from build123d import *

# Parameters (mm, degrees)
F1_DEPTH = 25
F3_DEPTH = 24


with BuildPart() as f1:
    # F0 (on Right) → F1 (new body)
    with BuildSketch(Plane.YZ):
        Polygon((0, 30.708406), (0, 0), (6.495294, 0), (6.495294, 8.168684), (15.046757, 8.168684), (15.046757, 14.439756), (6.637818, 14.439756), (6.637818, 21.7085), (46.972219, 21.7085), (46.972219, 0), (57.595324, 0), (57.595324, 30.708406), align=None)
    extrude(amount=F1_DEPTH)

    # F2 (on face) → F3 (cut)
    with BuildSketch(Plane(origin=(0, 0, 0), x_dir=(0, -1, 0), z_dir=(-1, 0, 0))):
        Polygon((-53.99179, -2.160003), (-53.99179, 28.144645), (-3.114748, 28.144645), (-3.114748, 0), (2.5671, 0), (2.5671, 33.474556), (-65.965217, 33.474556), (-65.965217, -2.160003), align=None)
    extrude(amount=-F3_DEPTH, mode=Mode.SUBTRACT)


solid = f1.part
Check sheet for the modelled part. Datum: model origin and axes. Units: mm. A direction names the side the tool comes from. Round coordinates to 2 decimals unless told otherwise and drop trailing zeros. Write each loop counter-clockwise with the first axis right and the second up, starting at its lowest first coordinate (ties: lowest second). Pieces come first, ordered by that corner, then holes. Notation, with made-up numbers: (-30.5, -33) - (-3.5, -33) arc R6 ccw to (-3.5, -25) - close; hole circle Ø5 at (-14, 78). An arc over 180 degrees is marked (long way). Return JSON: item names as keys, results as strings.
Q1. Depth check by flat-ended pin: P1, Ø4.5, axis at x = 17, y = 10.5, coming from the -Z side; P2, Ø8, axis at x = 17.5, z = 17.5, coming from the +Y side; P3, Ø11, axis at x = 18, z = 14, coming from the -Y side. Enter the tip coordinate at first touch or a pass-through.
Returned:
{"P1": "stops at z = 8.17", "P2": "stops at y = 53.99", "P3": "stops at y = 3.11"}
Q2. Cross-section at B-B (z = 5.5). Record the boundary of the cut face in (x, y).
Returned:
{"outline": "(0, 3.11) - (24, 3.11) - (24, 0) - (25, 0) - (25, 6.5) - (0, 6.5) - close; (0, 46.97) - (25, 46.97) - (25, 57.6) - (24, 57.6) - (24, 53.99) - (0, 53.99) - close"}
Q3. Cross-section at C-C (x = 3.5). Record the boundary of the cut face in (y, z).
Returned:
{"outline": "(3.11, 0) - (6.5, 0) - (6.5, 8.17) - (15.05, 8.17) - (15.05, 14.44) - (6.64, 14.44) - (6.64, 21.71) - (46.97, 21.71) - (46.97, 0) - (53.99, 0) - (53.99, 28.14) - (3.11, 28.14) - close"}
Q4. Draft check along Y on faces 1 (the flat face through (24, 35, 29)), 2 (the flat face through (12, 3.115, 14)), 3 (the flat face through (12, 27, 21.708)), 4 (the flat face through (12, 11, 8.169)). Enter one of: released by +Y, released by -Y, zero draft, split by the parting line, or undercut.
Returned:
{"face 1": "zero draft", "face 2": "released by -Y", "face 3": "undercut", "face 4": "undercut"}
Q5. Scan lines: L1, parallel to Y at x = 5.5, z = 21.5; L2, parallel to Y at x = 10, z = 9; L3, parallel to Z at x = 20.25, y = 8.5. Record each from-to range of solid material in increasing order. Write a range as from..to.
Returned:
{"L1": "y = 3.11..6.64, 46.97..53.99", "L2": "y = 3.11..15.05, 46.97..53.99", "L3": "z = 8.17..14.44, 21.71..28.14"}
Q6. Access from +Z, -Z, +X, -X, +Y, -Y to the whole of each face (thin tool, end or side, straight path). Record for faces 5 (the flat face through (12, 29, 28.145)), 6 (the flat face through (0, 28, 24)), 7 (the flat face through (12, 11, 14.44)), 8 (the flat face through (12, 53.992, 14)), 9 (the flat face through (12, 6.495, 4)).
Returned:
{"face 5": "+Z, -X, +Y, -Y", "face 6": "+Z, -Z, -X, +Y, -Y", "face 7": "+X, -X", "face 8": "+Z, -Z, -X, +Y", "face 9": "-Z, +X, -X"}
Q7. Cross-section at D-D (z = 24.5). Record the boundary of the cut face in (x, y), then the cut area to 3 significant figures.
Returned:
{"outline": "(0, 3.11) - (24, 3.11) - (24, 0) - (25, 0) - (25, 57.6) - (24, 57.6) - (24, 53.99) - (0, 53.99) - close", "area": "1,280 mm²"}
Q8. Cross-section at A-A (y = 12). Record the boundary of the cut face in (x, z), then the cut area to 3 significant figures.
Returned:
{"outline": "(0, 8.17) - (25, 8.17) - (25, 14.44) - (0, 14.44) - close; (0, 21.71) - (25, 21.71) - (25, 30.71) - (24, 30.71) - (24, 28.14) - (0, 28.14) - close", "area": "320 mm²"}
